Verification items for the finished model (mm, model axes). Face numbers are marked on the shaded views. A direction names the side the tool comes from. Coordinates: 2 decimals unless noted, no trailing zeros. Loops run counter-clockwise (first coordinate to the right, second up) from the corner with the lowest first, then second, coordinate; pieces in that order, holes last. Notation, with made-up numbers: (-23, 76.25) - (-16, 76.25) arc R16 ccw to (-16, 96.25) - close; hole circle Ø5 at (-37.5, -12). An arc over 180 degrees is marked (long way). One line per item, written item: value. Start each with the question number.
(1) Section check A-A (z = -19). Record the boundary of the cut face in (x, y) (1 decimal), plus the area to 3 significant figures.
(2) Gauge pin test, flat ends, axial feed: P1, Ø2, axis at x = -37, y = -23.5, coming from the +Z side; P2, Ø1.5, axis at y = -21.5, z = -1.5, coming from the -X side; P3, Ø4, axis at x = -94, z = -16, coming from the +Y side. Record the tip position at first contact, or that the pin passes through.
(3) Section check B-B (y = 4). Record the boundary of the cut face in (x, z).
(4) Set-up check for the marked faces 4 and 5: record each of +Z, -Z, +X, -X, +Y, -Y from which the full face is reachable in a straight line by a thin tool's end or side.
(5) Thickness scan on probe 1 along Z at (x, y) = (-32.5, -28); probe 2 along Y at (x, z) = (-23.5, -24.5); probe 3 along X at (y, z) = (21.5, -1.5). Record the ranges inside material, lowest first. Write a range as [from, to].
(6) Section check D-D (z = 0). Record the boundary of the cut face in (x, y), plus the area to 3 significant figures.
(7) Section check C-C (x = -110). Record the boundary of the cut face in (y, z), plus the area to 3 significant figures.
(8) Draft check along X on the marked faces 1, 2 and 3. Enter one of: +X half, -X half, draft (parallel to the pull), parting line (faces both ways), or undercut.
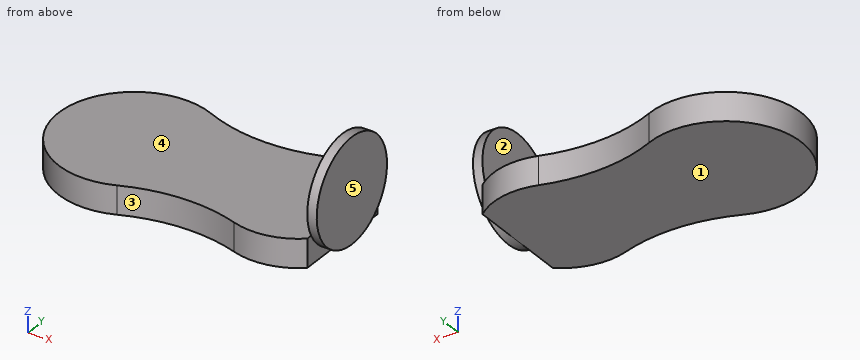
Autodesk Fusion 360 part; units mm, degrees
sketch "Sketch1" plane through (0, 0, 0) normal (1, 0, 0) x (0, 0, -1)
  circle A0 centre (0, 0) radius 27.5
  dimension "d1" = 55
extrude "Extrude1" add sketch "Sketch1" along normal blind 5
ref_plane "WorkPlane1" through (0, 0, -27.5) normal (0, 0, 1) x (1, 0, 0)
sketch "Sketch2" plane through (0, 0, -27.5) normal (0, 0, 1) x (1, 0, 0)
  line L0 (0, 0) -> (-150, 0)
  line L1 (0, 0) -> (-23, 0)
  line L2 (-150, 0) -> (-110, 0)
  line L3 (0, 0) -> (0, 27.5)
  circle A0 centre (-23, 0) radius 35.8504
  circle A1 centre (-110, 0) radius 40
  line L4 (0, 27.5) -> (0, -27.5)
  arc A2 (-94.2038, 36.7489) -> (-34.165, 34.0675) centre (-60.6369, 114.8402) ccw
  arc A3 (-34.165, -34.0675) -> (-94.2038, -36.7489) centre (-60.6369, -114.8402) ccw
  point P0 (0, -27.5)
  point P1 (0, 27.5)
  dimension "d6" = 150
  dimension "d7" = 23
  dimension "d8" = 40
  dimension "d9" = 27.5
  dimension "d10" = 85
extrude "Extrude2" add sketch "Sketch2" along normal blind 15 contours L0 L1 A0 L4 | L0 L1 L3 A0 L4 | L0 A0 A1 A3 | L0 A0 A1 A2 | L0 L2 A1 | L0 L2 A1
Responses:
1. outline: (-94.2, -36.7) arc R85 cw to (-34.2, -34.1) arc R35.9 ccw to (0, -27.5) - (0, -19.9) - (5, -19.9) - (5, 19.9) - (0, 19.9) - (0, 27.5) arc R35.9 ccw to (-34.2, 34.1) arc R85 cw to (-94.2, 36.7) arc R40 ccw (long way) to start
1. area: 10,100 mm²
2. P1: stops at z = -12.5
2. P2: stops at x = 0
2. P3: stops at y = 37.47
3. outline: (-149.8, -27.5) - (0, -27.5) - (0, -27.21) - (5, -27.21) - (5, 27.21) - (0, 27.21) - (0, -12.5) - (-149.8, -12.5) - close
4. face 4: +Z, -X, +Y, -Y
4. face 5: +Z, -Z, +X, +Y, -Y
5. probe 1: z = [-27.5, -12.5]
5. probe 2: y = [-35.85, 35.85]
5. probe 3: x = [0, 5]
6. outline: (0, -27.5) - (5, -27.5) - (5, 27.5) - (0, 27.5) - close
6. area: 275 mm²
7. outline: (-40, -27.5) - (40, -27.5) - (40, -12.5) - (-40, -12.5) - close
7. area: 1,200 mm²
8. face 1: draft
8. face 2: -X half
8. face 3: undercut
